The figure shows three views and two pictorial views of one solid part (mm, origin at its lowest corner). Answer the questions. A direction names the side the tool comes from. Give positions to 0.01 mm unless a question says otherwise; leave off trailing zeros. Order: outer loops, then holes, each group sorted by start corner. A loop starts at its lowest first (then second) coordinate and runs counter-clockwise, first axis right, second up. Notation, with made-up numbers: (50.5, -1.75) - (99.5, -1.75) arc R18 ccw to (99.5, 30.25) - close; hole circle Ø1 at (3.25, 46.25). An arc over 180 degrees is marked (long way). Answer as a JSON object with one key per item and string values. Group by question number.
Q1. Given pin 1 (10 mm diameter, centred on x = 23, z = 11.5, fed in from -Y); pin 2 (10 mm diameter, centred on x = 73, y = 20.5, fed in from +Z), each flat-ended and moving along its own axis, determine where each tip first touches the part or whether it passes through.
Q2. A cutting plane is placed at B-B, the plane z = 14.25. Give the vertices of the cut face in (x, y), and give its area (3 significant figures).
Q3. Consider line 1 (X direction, y = 53.5, z = 9.5); line 2 (Y direction, x = 32, z = 16.75); line 3 (Z direction, x = 89, y = 29). Determine where each line is inside the solid, lowest interval first.
Q4. A cutting plane is placed at C-C, the plane y = 23. Give the vertices of the cut face in (x, z), and give its area (3 significant figures).
Q5. A cutting plane is placed at A-A, the plane x = 88. Give the vertices of the cut face in (y, z), and give its area (4 significant figures).
Q6. For the marked faces 1 and 2, determine the directions among +Z, -Z, +X, -X, +Y, -Y from which every point of the face is accessible in a straight line to the end or side of a thin tool.
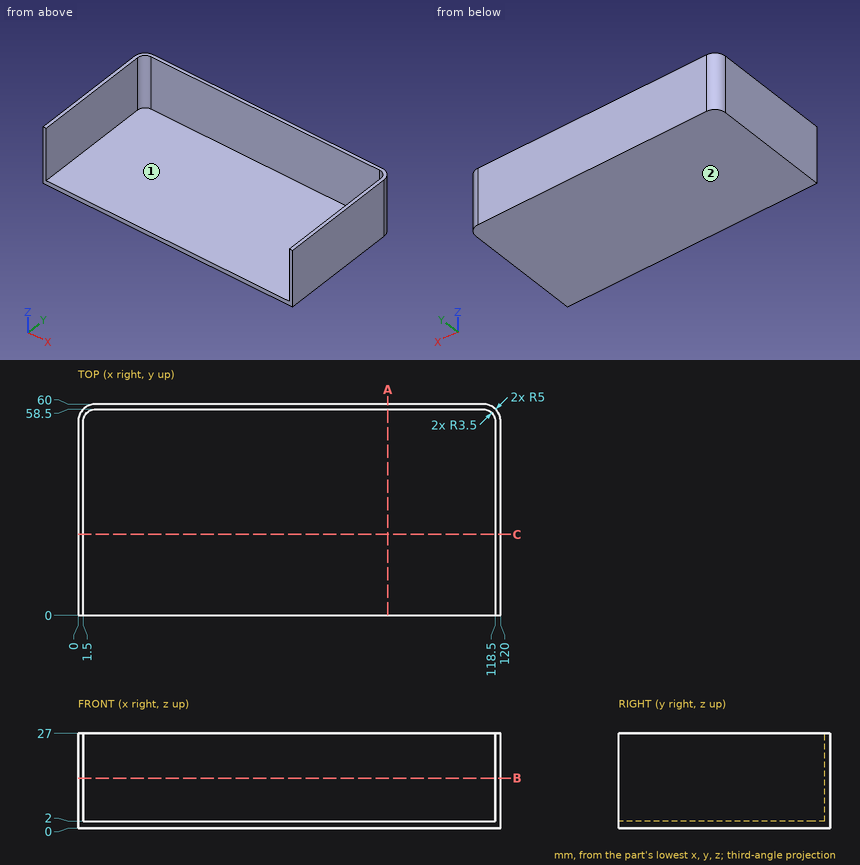
Reply:
{
 "1": {"pin 1": "stops at y = 58.5", "pin 2": "stops at z = 2"},
 "2": {"outline": "(0, 0) - (1.5, 0) - (1.5, 55) arc R3.5 cw to (5, 58.5) - (115, 58.5) arc R3.5 cw to (118.5, 55) - (118.5, 0) - (120, 0) - (120, 55) arc R5 ccw to (115, 60) - (5, 60) arc R5 ccw to (0, 55) - close", "area": "350 mm^2"},
 "3": {"line 1": "x = 0 to 1.5, 118.5 to 120", "line 2": "y = 58.5 to 60", "line 3": "z = 0 to 2"},
 "4": {"outline": "(0, 0) - (120, 0) - (120, 27) - (118.5, 27) - (118.5, 2) - (1.5, 2) - (1.5, 27) - (0, 27) - close", "area": "315 mm^2"},
 "5": {"outline": "(0, 0) - (60, 0) - (60, 27) - (58.5, 27) - (58.5, 2) - (0, 2) - close", "area": "157.5 mm^2"},
 "6": {"face 1": "+Z, -Y", "face 2": "-Z, +X, -X, +Y, -Y"}
}
